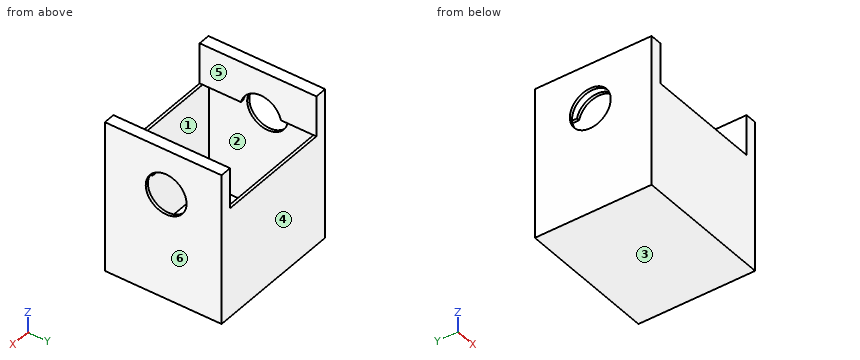
from build123d import *

# Parameters (mm, degrees)
F0_W     = 120
F0_H     = 130
F1_DEPTH = 100
F2_W     = 100
F2_H     = 35
F3_DEPTH = 125
F4_T     = -2.5
F5_R     = 17.5
F6_DEPTH = 5005


# Not quite as in the source:
# - a shell that OpenCascade refuses in one call is made with other operations: the cavity is built on its own and cut out


with BuildPart() as f1:
    # F0 (on Front) → F1 (new body)
    with BuildSketch(Plane.XZ):
        with Locations((-0.7081851363, 2.2362722828)):
            Rectangle(F0_W, F0_H)
    extrude(amount=F1_DEPTH)

    # F2 (on face) → F3 (cut)
    with BuildSketch(Plane.XZ.offset(100)):
        with Locations((-0.5643002689, 49.7362722828)):
            Rectangle(F2_W, F2_H)
    extrude(amount=-F3_DEPTH, mode=Mode.SUBTRACT)

    # F4: a shell. OpenCascade refuses it in one call, so the cavity is built on its own and cut out:
    # the body offset inwards by the wall thickness, plus a prism from it out through each open face.
    f4_core = offset(f1.part, amount=F4_T, kind=Kind.INTERSECTION, mode=Mode.PRIVATE)
    f4_exits = [f4_core.faces().sort_by_distance(p)[0] for p in [
        (-0.5643, -50, 29.736272),
    ]]
    add(f4_core, mode=Mode.SUBTRACT)
    extrude(f4_exits, amount=-F4_T, mode=Mode.SUBTRACT)

    # F5 (on face) → F6 (cut)
    with BuildSketch(Plane(origin=(-60.7081851363, 0, 0), x_dir=(0, -1, 0), z_dir=(-1, 0, 0))):
        with Locations((47.4842637777, 28.4689757973)):
            Circle(F5_R)
    extrude(amount=-F6_DEPTH, mode=Mode.SUBTRACT)


solid = f1.part
Read the model definition and answer for the solid it produces. Units are mm, in the model's axes. Face numbers are marked on the shaded views. A direction names the side the tool comes from. Give positions to 0.01 mm unless a question says otherwise; leave off trailing zeros. Write each loop counter-clockwise with the first axis right and the second up, starting at its lowest first coordinate (ties: lowest second). Pieces come first, ordered by that corner, then holes. Notation, with made-up numbers: (12, -28.5) -> (67, -28.5) arc R21 cw to (67, -20.5) -> close; hole circle Ø6 at (75.25, 44). An arc over 180 degrees is marked (long way). Answer as a JSON object with one key per item and string values. Group by question number.
1) A tool of negligible diameter and unlimited length cuts with its end or side. For the marked faces 5 and 6, from which of +Z, -Z, +X, -X, +Y, -Y can it reach the whole face along a straight path? Write none if from no direction.
2) Find section A-A (z = 9). Write down the section's boundary in (x, y).
3) Find section D-D (y = -11.5). Write down the section's boundary in (x, z).
4) Each of these flat-tipped pins is pushed along its axis until it touches: P1, Ø1.2, axis at x = -13, y = -1, coming from the +Z side; P2, Ø1, axis at x = -5.5, y = -15, coming from the +Z side. Where does it stop, or does it pass through?
5) Find section B-B (y = -58). Write down the section's boundary in (x, z), and give its area (3 significant figures).
6) Consider L1, parallel to X at y = -40, z = 49; L2, parallel to X at y = -35.5, z = 9; L3, parallel to Y at x = 53, z = 32.5. Determine where each line is inside the solid, lowest interval first. Write a range as from..to.
7) Find section C-C (x = 47). Write down the section's boundary in (y, z), and give its area (4 significant figures).
8) The mould has two halves that part along Z. Classify the marked faces 1, 2, 3 and 4: +Z half, -Z half, draft (parallel to the pull), parting line (faces both ways), or undercut.
Values follow:
{
 "1": {"face 5": "+Z, +Y, -Y", "face 6": "+Z, -Z, +X, +Y, -Y"},
 "2": {"outline": "(-60.71, -100) -> (59.29, -100) -> (59.29, 0) -> (-60.71, 0) -> close; hole (-58.21, -97.5) -> (56.79, -97.5) -> (56.79, -2.5) -> (-58.21, -2.5) -> close"},
 "3": {"outline": "(-60.71, -62.76) -> (59.29, -62.76) -> (59.29, 67.24) -> (49.44, 67.24) -> (49.44, 32.24) -> (51.94, 32.24) -> (51.94, 64.74) -> (56.79, 64.74) -> (56.79, -60.26) -> (-58.21, -60.26) -> (-58.21, 64.74) -> (-53.06, 64.74) -> (-53.06, 32.24) -> (-50.56, 32.24) -> (-50.56, 67.24) -> (-60.71, 67.24) -> close"},
 "4": {"P1": "stops at z = 32.24", "P2": "stops at z = -60.26"},
 "5": {"outline": "(-60.71, -62.76) -> (59.29, -62.76) -> (59.29, 14.48) -> (56.79, 14.48) -> (56.79, -60.26) -> (-58.21, -60.26) -> (-58.21, 14.48) -> (-60.71, 14.48) -> close; (-60.71, 42.46) -> (-58.21, 42.46) -> (-58.21, 64.74) -> (-53.06, 64.74) -> (-53.06, 42.46) -> (-50.56, 42.46) -> (-50.56, 67.24) -> (-60.71, 67.24) -> close; (49.44, 42.46) -> (51.94, 42.46) -> (51.94, 64.74) -> (56.79, 64.74) -> (56.79, 42.46) -> (59.29, 42.46) -> (59.29, 67.24) -> (49.44, 67.24) -> close", "area": "947 mm2"},
 "6": {"L1": "x = -60.71..-58.21, -53.06..-50.56, 49.44..51.94, 56.79..59.29", "L2": "x = -60.71..-58.21, 56.79..59.29", "L3": "y = -100..-97.5, -2.5..0"},
 "7": {"outline": "(-100, -62.76) -> (0, -62.76) -> (0, 32.24) -> (-2.5, 32.24) -> (-2.5, -60.26) -> (-97.5, -60.26) -> (-97.5, 32.24) -> (-100, 32.24) -> close", "area": "712.5 mm2"},
 "8": {"face 1": "undercut", "face 2": "undercut", "face 3": "-Z half", "face 4": "draft"}
}
